The model under review builds one solid part; all positions refer to its coordinate system, in mm. A direction names the side the tool comes from. Round coordinates to 2 decimals unless told otherwise and drop trailing zeros. Order: outer loops, then holes, each group sorted by start corner. A loop starts at its lowest first (then second) coordinate and runs counter-clockwise, first axis right, second up. Notation, with made-up numbers: (61.5, -16) -> (120.5, -16) arc R14 cw to (120.5, 7) -> close; hole circle Ø3 at (-31, 0.25). An arc over 180 degrees is marked (long way). Use a Markdown table: item, result. Add a question column.
```python
from build123d import *

# Parameters (mm, degrees)
F0_R     = 5
F1_DEPTH = 400
F2_W     = 10
F2_H     = 10
F3_DEPTH = 10
F4_R     = 2.5
F5_DEPTH = 25


with BuildPart() as f1:
    # F0 (on Right) → F1 (new body)
    with BuildSketch(Plane.YZ):
        Circle(F0_R)
    extrude(amount=F1_DEPTH)

    # F2 (on face) → F3 (join)
    with BuildSketch(Plane(origin=(0, 0, 0), x_dir=(0, -1, 0), z_dir=(-1, 0, 0))):
        Rectangle(F2_W, F2_H)
    extrude(amount=F3_DEPTH)

    # F4 (on face) → F5 (cut)
    with BuildSketch(Plane.XZ.offset(5)):
        with Locations((-5, 0)):
            Circle(F4_R)
    extrude(amount=-F5_DEPTH, mode=Mode.SUBTRACT)


solid = f1.part
```
Q1. Add section B-B, the plane x = 225.5. Give the boundary of the cut face in (y, z), then the cut area to 3 significant figures.
Q2. For pin 1 (2 mm diameter, centred on x = 60.5, z = 2, fed in from -Y); pin 2 (1.5 mm diameter, centred on x = 236, z = 2, fed in from +Y), all flat-tipped, find the tip position at first contact; note any pin that passes through.
Q3. Add section A-A, the plane y = -3. Give the boundary of the cut face in (x, z).
Q4. For faces 1 (the face through (400, 0, 0)), 2 (the face through (197.2, -1.08, -4.88)), list the 3-axis set-ups (+Z, -Z, +X, -X, +Y, -Y) from which the entire face can be reached by the end or side of a thin tool; tool diameter is ignored.
Q5. To check wall thickness, follow line 1 along Z through (x, y) = (-5, -0.5); line 2 along Z through (x, y) = (65, -0.5); line 3 along Y through (x, z) = (295.5, 0.75). State the ranges of each line that lie inside material, in increasing order.
Return value:
| question | item | result |
|---|---|---|
| 1 | outline | circle Ø10 at (0, 0) |
| 1 | area | 78.5 mm² |
| 2 | pin 1 | y = -4.9 |
| 2 | pin 2 | y = 4.84 |
| 3 | outline | (-10, -5) -> (0, -5) -> (0, -4) -> (400, -4) -> (400, 4) -> (0, 4) -> (0, 5) -> (-10, 5) -> close; hole circle Ø5 at (-5, 0) |
| 4 | face 1 | +Z, -Z, +X, +Y, -Y |
| 4 | face 2 | +X |
| 5 | line 1 | -5 to -2.5, 2.5 to 5 |
| 5 | line 2 | -4.97 to 4.97 |
| 5 | line 3 | -4.94 to 4.94 |
